Autodesk Inventor part; units mm, degrees
ref_plane "Work Plane5" through (-20.32, 0, 18.3236) normal (0, 0, 1) x (1, 0, 0)
ref_plane "Work Plane4" through (-20.32, 0, 18.3236) normal (0, 0, 1) x (1, 0, 0)
ref_plane "Work Plane2" through (-20.32, 0, 18.3236) normal (0, 0, 1) x (1, 0, 0)
sketch "Sketch1" plane through (0, 0, 0) normal (0, 1, 0) x (-1, 0, 0)
  line L0 (-20.32, 15.1384) -> (-20.32, -15.1384)
  line L1 (-20.32, -15.1384) -> (20.32, -15.1384)
  line L2 (20.32, -15.1384) -> (20.32, 15.1384)
  line L3 (20.32, 15.1384) -> (-20.32, -15.1384) construction
  line L4 (-20.32, 15.1384) -> (20.32, -15.1384) construction
  line L5 (20.32, 15.1384) -> (-20.32, 15.1384)
  point P0 (0, 0)
  dimension "d9" = 30.2768
  dimension "d23" = 40.64
extrude "Extrusion1" add sketch "Sketch1" along normal blind 6.35
sketch "Sketch3" plane through (-20.32, 0, 15.1384) normal (0, 0, 1) x (1, 0, 0)
  point P0 (20.32, 0)
  point P1 (0, 0)
sketch "Sketch4" plane through (20.32, 0, -15.1384) normal (0, 0, -1) x (-1, 0, 0)
  line L0 (0, 0) -> (0, 6.35)
  line L1 (0, 6.35) -> (12.418, 15.828)
  line L2 (40.64, 0) -> (40.64, 6.35)
  line L3 (40.64, 6.35) -> (16.6386, 16.372)
  arc A0 (16.6386, 16.372) -> (12.418, 15.828) centre (14.9993, 12.446) ccw
  line L4 (40.64, 0) -> (0, 0)
  circle A1 centre (14.9993, 12.446) radius 1.7145
  circle A2 centre (14.9993, 12.446) radius 2.4511
  point P0 (20.32, 0)
  dimension "d14" = 3.429
  dimension "d24" = 2.54
ref_plane "Work Plane5" through (-20.32, 0, 18.3236) normal (0, 0, 1) x (1, 0, 0)
extrude "Extrusion6" add sketch "Sketch4" along normal blind 3.175 contours L0 L1 A0 L3 L2 L4 | A2
sketch "Sketch6" plane through (0, 6.35, 0) normal (0, 1, 0) x (1, 0, 0)
  circle A0 centre (-4.1879, -9.9736) radius 1.05
  circle A1 centre (8.3121, -9.9736) radius 1.05
  circle A2 centre (8.3121, 11.0264) radius 1.05
  circle A3 centre (-4.1879, 11.0264) radius 1.05
  point P0 (0, 0)
extrude "Extrusion7" cut sketch "Sketch6" against normal up to next
ref_plane "Work Plane4" through (-20.32, 0, 18.3236) normal (0, 0, 1) x (1, 0, 0)
sketch "Sketch13" plane through (0, 6.35, 0) normal (0, 1, 0) x (1, 0, 0)
  circle A0 centre (-4.1879, 11.0264) radius 1.05
  line L0 (-2.0289, 9.7799) -> (-4.1879, 8.5334)
  line L1 (-4.1879, 8.5334) -> (-6.3469, 9.7799)
  line L2 (-6.3469, 9.7799) -> (-6.3469, 12.2729)
  line L3 (-6.3469, 12.2729) -> (-4.1879, 13.5194)
  line L4 (-4.1879, 13.5194) -> (-2.0289, 12.2729)
  line L5 (-2.0289, 12.2729) -> (-2.0289, 9.7799)
  circle A1 centre (8.3121, 11.0264) radius 1.05
  line L6 (10.4711, 9.7799) -> (8.3121, 8.5334)
  line L7 (8.3121, 8.5334) -> (6.1531, 9.7799)
  line L8 (6.1531, 9.7799) -> (6.1531, 12.2729)
  line L9 (6.1531, 12.2729) -> (8.3121, 13.5194)
  line L10 (8.3121, 13.5194) -> (10.4711, 12.2729)
  line L11 (10.4711, 12.2729) -> (10.4711, 9.7799)
  circle A2 centre (-4.1879, -9.9736) radius 1.05
  line L12 (-2.0289, -11.2201) -> (-4.1879, -12.4666)
  line L13 (-4.1879, -12.4666) -> (-6.3469, -11.2201)
  line L14 (-6.3469, -11.2201) -> (-6.3469, -8.7271)
  line L15 (-6.3469, -8.7271) -> (-4.1879, -7.4806)
  line L16 (-4.1879, -7.4806) -> (-2.0289, -8.7271)
  line L17 (-2.0289, -8.7271) -> (-2.0289, -11.2201)
  circle A3 centre (8.3121, -9.9736) radius 1.05
  line L18 (10.4711, -11.2201) -> (8.3121, -12.4666)
  line L19 (8.3121, -12.4666) -> (6.1531, -11.2201)
  line L20 (6.1531, -11.2201) -> (6.1531, -8.7271)
  line L21 (6.1531, -8.7271) -> (8.3121, -7.4806)
  line L22 (8.3121, -7.4806) -> (10.4711, -8.7271)
  line L23 (10.4711, -8.7271) -> (10.4711, -11.2201)
  line L24 (-20.32, 15.1384) -> (-20.32, -15.1384)
  circle A4 centre (0, 0) radius 1.7967
extrude "Extrusion12" cut sketch "Sketch13" against normal blind 2.9972 contours L0 L1 L2 L3 L4 L5 | L6 L7 L8 L9 L10 L11 | L12 L13 L14 L15 L16 L17 | L18 L19 L20 L21 L22 L23
ref_plane "Work Plane2" through (-20.32, 0, 18.3236) normal (0, 0, 1) x (1, 0, 0)
ref_plane "Work Plane7" through (-20.32, 0, -1.5875) normal (0, 0, 1) x (1, 0, 0)
sketch "Sketch17" plane through (-20.32, 0, 15.1384) normal (0, 0, 1) x (1, 0, 0)
  line L0 (0, 0) -> (0, 6.35)
  line L1 (40.64, 6.35) -> (0, 6.35)
  line L2 (0, 0) -> (40.64, 0)
  line L3 (40.64, 0) -> (40.64, 6.35)
  line L4 (40.64, 6.35) -> (0, 6.35)
  line L5 (0, 6.35) -> (0, 0)
  point P0 (20.32, 0)
extrude "Extrusion16" add sketch "Sketch17" along normal blind 1
ref_plane "Work Plane9" through (-20.32, 0, -1.0877) normal (0, 0, 1) x (1, 0, 0)
mirror "Mirror2" about plane through (-20.32, 0, -1.0877) normal (0, 0, 1) of "Extrusion6"
properties part number "CameraMount" material "ABS Plastic"
The listing builds one solid part. Answer for the finished solid, in the listing's coordinates (mm). A direction names the side the tool comes from. Give positions to 0.01 mm unless a question says otherwise; leave off trailing zeros. Order: outer loops, then holes, each group sorted by start corner. A loop starts at its lowest first (then second) coordinate and runs counter-clockwise, first axis right, second up. Notation, with made-up numbers: (88.5, -19) - (131.5, -19) arc R29 ccw to (131.5, 18) - close; hole circle Ø4 at (54.25, -20). An arc over 180 degrees is marked (long way). One line per item, written item: value. Start each with the question number.
1) The mould has two halves that part along Y. Classify faces 1 (the face through (-5.28, 4.87, -12.89)), 2 (the face through (6.68, 13.49, -16.7)), 3 (the face through (6.584, 13.605, 14.528)), 4 (the face through (-5, 3.353, -10)): released by +Y, released by -Y, zero draft, split by the parting line, or undercut.
2) A cutting plane is placed at C-C on y = 8. Give the vertices of the cut face in (x, z), then the cut area to 3 significant figures.
3) A cutting plane is placed at B-B on z = -10.5. Give the vertices of the cut face in (x, y), then the cut area to 3 significant figures.
4) A tool of negligible diameter and unlimited length cuts with its end or side. For faces 5 (the face through (-4.4, 1.7, -10)), 6 (the face through (-5, 5, -9)), from which of +Z, -Z, +X, -X, +Y, -Y can it reach the whole face along a straight path? Write none if from no direction.
5) Find the intervals of material crossed by L1, parallel to X at y = 6.25, z = 9; L2, parallel to Z at x = 2, y = 9.25; L3, parallel to X at y = 2.25, z = -11.5, in increasing order.
6) Given pin 1 Ø1.3 at (x, z) = (9, -11) entering from +Y; pin 2 Ø3.5 at (x, z) = (7.5, 10) entering from +Y; pin 3 Ø1.9 at (x, z) = (8.31, 9.97) entering from -Y, each flat-ended and moving along its own axis, determine where each tip first touches the part or whether it passes through.
7) A cutting plane is placed at A-A on y = 4. Give the vertices of the cut face in (x, z).
Answer sheet:
1. face 1: zero draft
1. face 2: undercut
1. face 3: undercut
1. face 4: released by +Y
2. outline: (-16.37, -18.31) - (18.16, -18.31) - (18.16, -15.14) - (-16.37, -15.14) - close; (-16.37, 12.96) - (18.16, 12.96) - (18.16, 16.14) - (-16.37, 16.14) - close
2. area: 219 mm2
3. outline: (-20.32, 0) - (-5.1, 0) - (-5.1, 3.35) - (-6.35, 3.35) - (-6.35, 6.35) - (-20.32, 6.35) - close; (-3.28, 0) - (7.4, 0) - (7.4, 3.35) - (6.15, 3.35) - (6.15, 6.35) - (-2.03, 6.35) - (-2.03, 3.35) - (-3.28, 3.35) - close; (9.22, 0) - (20.32, 0) - (20.32, 6.35) - (10.47, 6.35) - (10.47, 3.35) - (9.22, 3.35) - close
3. area: 220 mm2
4. face 5: +Y, -Y
4. face 6: +Y
5. L1: x = -20.32 to -6.35, -2.03 to 6.15, 10.47 to 20.32
5. L2: z = -18.31 to -15.14, 12.96 to 16.14
5. L3: x = -20.32 to -5.13, -3.25 to 7.37, 9.25 to 20.32
6. pin 1: stops at y = 3.35
6. pin 2: stops at y = 6.35
6. pin 3: passes through
7. outline: (-20.32, -18.31) - (20.32, -18.31) - (20.32, 16.14) - (-20.32, 16.14) - close; hole (-6.35, -12.27) - (-4.19, -13.52) - (-2.03, -12.27) - (-2.03, -9.78) - (-4.19, -8.53) - (-6.35, -9.78) - close; hole (-6.35, 8.73) - (-4.19, 7.48) - (-2.03, 8.73) - (-2.03, 11.22) - (-4.19, 12.47) - (-6.35, 11.22) - close; hole (6.15, -12.27) - (8.31, -13.52) - (10.47, -12.27) - (10.47, -9.78) - (8.31, -8.53) - (6.15, -9.78) - close; hole (6.15, 8.73) - (8.31, 7.48) - (10.47, 8.73) - (10.47, 11.22) - (8.31, 12.47) - (6.15, 11.22) - close
